```python
from build123d import *

# Parameters (mm, degrees)
SKETCH_1_R               = 6
SKETCH_1_R_2             = 4
EXTRUDE_1_DEPTH          = 15
CUT_EXTRUDE_1_DEPTH      = 18.23368794
CUT_EXTRUDE_1_DEPTH_BACK = 18.23368794
FILLET_1_R               = 0.3


with BuildPart() as part:
    # Эскиз1 → Бобышка-Вытянуть1 (new body)
    with BuildSketch(Plane(origin=(0, 0, 0), x_dir=(1, 0, 0), z_dir=(0, 1, 0))):
        with Locations(Location((0, 0, 0), (0, 0, 270))):
            Circle(SKETCH_1_R)
        with Locations(Location((0, 0, 0), (0, 0, 270))):
            Circle(SKETCH_1_R_2, mode=Mode.SUBTRACT)
    extrude(amount=EXTRUDE_1_DEPTH)

    # Эскиз2 → Вырез-Вытянуть1 (cut, two sides: drawn at the far end of the back side and taken through both)
    with BuildSketch(Plane.XY.offset(-CUT_EXTRUDE_1_DEPTH_BACK)):
        with BuildLine():
            Line((5, 14), (2.828427125, 11.828427125))
            ThreePointArc((2.828427125, 11.828427125), (0, 10.656854249), (-2.828427125, 11.828427125))
            Line((-2.828427125, 11.828427125), (-5, 14))
            Line((-5, 14), (-7.91663408, 14))
            Line((-7.91663408, 14), (-7.91663408, 18.742378879))
            Line((-7.91663408, 18.742378879), (8.078053183, 18.742378879))
            Line((8.078053183, 18.742378879), (8.078053183, 14))
            Line((8.078053183, 14), (5, 14))
        make_face()
    extrude(amount=CUT_EXTRUDE_1_DEPTH + CUT_EXTRUDE_1_DEPTH_BACK, mode=Mode.SUBTRACT)

    # Скругление1
    fillet_1_edges = [part.edges().sort_by_distance(p)[0] for p in [
        (0, 0, -6),
    ]]
    fillet(fillet_1_edges, radius=FILLET_1_R)


solid = part.part
```
Could you check a few things on this model? Use its own coordinates, in mm. A direction names the side the tool comes from. Round coordinates to 2 decimals unless told otherwise and drop trailing zeros. Loops run counter-clockwise (first coordinate to the right, second up) from the corner with the lowest first, then second, coordinate; pieces in that order, holes last. Notation, with made-up numbers: M 40,-33 L 97,-33 A14 cw 97,-26 Z; hole C 33.25,8 d1. An arc over 180 degrees is marked long. Put each result on its own line as item: value.
Q1. Imagine slicing it at B-B (z = 0). Write out the boundary of the cut face in (x, y).
Check result:
outline: M -6,0.3 A0.3 ccw -5.7,0 L -4,0 L -4,13 L -5,14 L -6,14 Z; M 4,0 L 5.7,0 A0.3 ccw 6,0.3 L 6,14 L 5,14 L 4,13 Z
Q2. Imagine slicing it at D-D (y = 9). Write out the boundary of the cut face in (x, z), then the cut area to 3 significant figures.
Check result:
outline: C 0,0 d12; hole C 0,0 d8
area: 62.8 mm2
Q3. Thinking about a two-plate mould opening in X: for faces 1 (the face through (0, 7, -6)), 2 (the face through (-4.14, 13.14, -0.07)), 3 (the face through (-5.4, 14, 0)), which applies, released by +X, released by -X, zero draft, split by the parting line, or undercut?
Check result:
face 1: split by the parting line
face 2: undercut
face 3: zero draft
Q4. On a 3-axis mill with a long thin cutter (end or side, diameter ignored), from which of +Z, -Z, +X, -X, +Y, -Y can I reach the whole of each face in a straight line? I mean faces 4 (the face through (-4, 0, 2)), 5 (the face through (4.2, 13.2, -0.1)). Say none if no direction works.
Check result:
face 4: +Z, -Z, +X, -X, -Y
face 5: +Z, -Z, +Y
Q5. I need wall thicknesses on probe 1 along X at (y, z) = (3.5, 0); probe 2 along X at (y, z) = (12.75, -2). Which ranges of each line are inside material? Lowest first, please.
Check result:
probe 1: -6 to -4, 4 to 6
probe 2: -5.66 to -3.75, 3.75 to 5.66
Q6. Imagine slicing it at C-C (y = 12.75). Write out the boundary of the cut face in (x, z), then the cut area to 3 significant figures.
Check result:
outline: M -3.75,-4.68 L -3.75,-1.39 A4 cw -3.75,1.39 L -3.75,4.68 A6 ccw Z; M 3.75,-4.68 A6 ccw 3.75,4.68 L 3.75,1.39 A4 cw 3.75,-1.39 Z
area: 28.4 mm2
Q7. For pin 1 (2 mm diameter, centred on y = 2, z = 3.5, fed in from -X); pin 2 (1.5 mm diameter, centred on x = -4, y = 1.5, fed in from -Z); pin 3 (6 mm diameter, centred on x = 4, y = 4, fed in from +Z), each with a flat end and sliding along its axis, tell me the tip position at first contact or that it passes through.
Check result:
pin 1: x = -5.45
pin 2: z = -5.04
pin 3: z = 5.92
Q8. Imagine slicing it at A-A (x = 0). Write out the boundary of the cut face in (y, z).
Check result:
outline: M 0,-5.7 A0.3 ccw 0.3,-6 L 10.66,-6 L 10.66,-4 L 0,-4 Z; M 0,4 L 10.66,4 L 10.66,6 L 0.3,6 A0.3 ccw 0,5.7 Z
